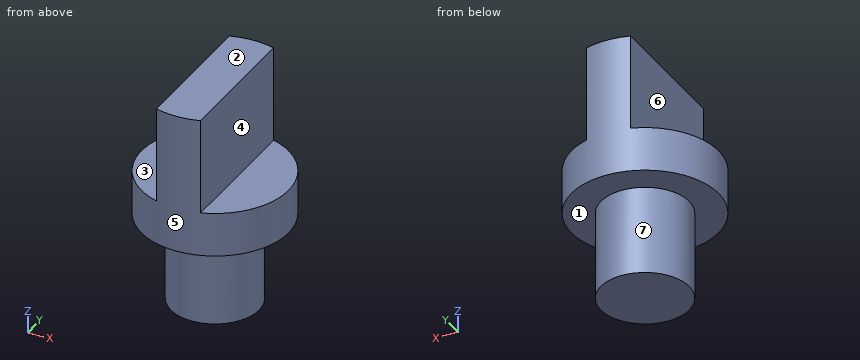
```python
from build123d import *

# Parameters (mm, degrees)
F0_R     = 10
F1_DEPTH = 31
F3_DEPTH = 13
F4_R     = 10
F4_R_2   = 6
F5_DEPTH = 12


with BuildPart() as f1:
    # F0 (on Top) → F1 (new body)
    with BuildSketch(Plane.XY):
        Circle(F0_R)
    extrude(amount=F1_DEPTH)

    # F2 (on face) → F3 (cut)
    with BuildSketch(Plane.XY.offset(31)):
        with BuildLine():
            Line((3, 9.5393920142), (3, 0))
            Line((3, 0), (3, -9.5393920142))
            ThreePointArc((3, -9.5393920142), (8.0622577483, -5.9160797831), (10, 0))
            ThreePointArc((10, 0), (8.0622577483, 5.9160797831), (3, 9.5393920142))
        make_face()
        with BuildLine():
            Line((-3, -9.5393920142), (-3, 0))
            Line((-3, 0), (-3, 9.5393920142))
            ThreePointArc((-3, 9.5393920142), (-10, 0), (-3, -9.5393920142))
        make_face()
    extrude(amount=-F3_DEPTH, mode=Mode.SUBTRACT)

    # F4 (on face) → F5 (cut)
    with BuildSketch(Plane(origin=(0, 0, 0), x_dir=(1, 0, 0), z_dir=(0, 0, -1))):
        Circle(F4_R)
        Circle(F4_R_2, mode=Mode.SUBTRACT)
    extrude(amount=-F5_DEPTH, mode=Mode.SUBTRACT)


solid = f1.part
```
For this review, take the finished solid that the model builds, in its own axes (mm). Face numbers are marked on the shaded views. A direction names the side the tool comes from. Coordinates: 2 decimals unless noted, no trailing zeros. Loops run counter-clockwise (first coordinate to the right, second up) from the corner with the lowest first, then second, coordinate; pieces in that order, holes last.
1. Add section D-D, the plane y = 3.5. Give the boundary of the cut face in (x, z), then the cut area to 3 significant figures.
2. Add section B-B, the plane x = 0. Give the boundary of the cut face in (y, z), then the cut area to 3 significant figures.
3. Add section A-A, the plane y = 0. Give the boundary of the cut face in (x, z).
4. Insertion check: P1, Ø5, axis at x = 7, y = 1, coming from the +Z side; P2, Ø6.5, axis at y = 4, z = 23.5, coming from the +X side; P3, Ø10, axis at y = -0.5, z = 3.5, coming from the -X side. Each pin has a flat end and moves straight along its axis. Give the tip position at first contact, or say it passes through.
5. Add section C-C, the plane z = 25. Give the boundary of the cut face in (x, y).
6. Mouldability with a two-part tool opening along Y and no side actions: class the marked faces 6 and 7 as +Y half, -Y half, draft (parallel to the pull), parting line (faces both ways), or undercut.
7. For the marked faces 1, 2, 3, 4 and 5, list the 3-axis set-ups (+Z, -Z, +X, -X, +Y, -Y) from which the entire face can be reached by the end or side of a thin tool; tool diameter is ignored.
8. For line 1 (Z direction, x = -4, y = 3.5); line 2 (Z direction, x = -1.5, y = -6); line 3 (X direction, y = 6.75, z = 20.5), list the stretches that pass through material, from the lowest coordinate up.
Result:
1. outline: (-9.37, 12) - (-4.87, 12) - (-4.87, 0) - (4.87, 0) - (4.87, 12) - (9.37, 12) - (9.37, 18) - (3, 18) - (3, 31) - (-3, 31) - (-3, 18) - (-9.37, 18) - close
1. area: 307 mm2
2. outline: (-10, 12) - (-6, 12) - (-6, 0) - (6, 0) - (6, 12) - (10, 12) - (10, 31) - (-10, 31) - close
2. area: 524 mm2
3. outline: (-10, 12) - (-6, 12) - (-6, 0) - (6, 0) - (6, 12) - (10, 12) - (10, 18) - (3, 18) - (3, 31) - (-3, 31) - (-3, 18) - (-10, 18) - close
4. P1: stops at z = 18
4. P2: stops at x = 3
4. P3: stops at x = -6
5. outline: (-3, -9.54) arc R10 ccw to (3, -9.54) - (3, 9.54) arc R10 ccw to (-3, 9.54) - close
6. face 6: draft
6. face 7: parting line
7. face 1: -Z
7. face 2: +Z, +X, -X, +Y, -Y
7. face 3: +Z, -X, +Y, -Y
7. face 4: +Z, +X, +Y, -Y
7. face 5: +Z, -Z
8. line 1: z = 0 to 18
8. line 2: z = 12 to 31
8. line 3: x = -3 to 3
